Verification items for the finished model (mm, model axes). A direction names the side the tool comes from. Round coordinates to 2 decimals unless told otherwise and drop trailing zeros. Write each loop counter-clockwise with the first axis right and the second up, starting at its lowest first coordinate (ties: lowest second). Pieces come first, ordered by that corner, then holes. Notation, with made-up numbers: (40.25, -40) - (92.25, -40) arc R13 ccw to (92.25, -16) - close; hole circle Ø11 at (-38, -31). An arc over 180 degrees is marked (long way). Answer as a JSON object with one key per item and string values.
Autodesk Inventor part; units mm, degrees
ref_plane "YZ Plane" through (0, 0, 0) normal (1, 0, 0) x (0, 1, 0)
ref_plane "XZ Plane" through (0, 0, 0) normal (0, 1, 0) x (-1, 0, 0)
ref_plane "XY Plane" through (0, 0, 0) normal (0, 0, 1) x (1, 0, 0)
sketch "Sketch1" plane through (0, 0, 0) normal (0, 0, 1) x (1, 0, 0)
  arc A0 (6.3048, 12.5) -> (6.3048, -12.5) centre (0, 0) ccw
  arc A1 (193.6952, -12.5) -> (193.6952, 12.5) centre (200, 0) ccw
  line L0 (6.3048, 12.5) -> (193.6952, 12.5)
  line L1 (193.6952, -12.5) -> (6.3048, -12.5)
  dimension "d0" = 25
  dimension "d2" = 14
  dimension "d3" = 200
extrude "Extrusion1" add sketch "Sketch1" along normal blind 25
sketch "Sketch2" plane through (0, 0, 25) normal (0, 0, 1) x (1, 0, 0)
  arc A0 (6.3048, 12.5) -> (6.3048, -12.5) centre (0, 0) ccw
  arc A1 (193.6952, -12.5) -> (193.6952, 12.5) centre (200, 0) ccw
  circle A2 centre (0, 0) radius 11.05
  circle A3 centre (200, 0) radius 11.05
  dimension "d6" = 22.1
extrude "Extrusion2" cut sketch "Sketch2" against normal blind 7
sketch "Sketch3" plane through (0, 0, 0) normal (0, 0, -1) x (-1, 0, 0)
  circle A0 centre (-200, 0) radius 11.05
  circle A1 centre (0, 0) radius 11.05
extrude "Extrusion3" cut sketch "Sketch3" against normal blind 7
sketch "Sketch4" plane through (200, 0, 7) normal (0, 0, -1) x (-1, 0, 0)
  circle A0 centre (0, 0) radius 11.05
  circle A1 centre (200, 0) radius 11.05
  circle A2 centre (0, 0) radius 7.55
  circle A3 centre (200, 0) radius 7.55
  dimension "d12" = 15.1
extrude "Extrusion4" cut sketch "Sketch4" against normal through all contours A2 | A3
chamfer "Chamfer1" distance 3.5 angle 45 2 edges at (207.55, 0, 7) (7.55, 0, 7)
properties part number "ARM"
1. Cross-section at D-D (z = 13.75). Record the boundary of the cut face in (x, y), plus the area to 3 significant figures.
Completed:
{"outline": "(6.3, -12.5) - (193.7, -12.5) arc R14 ccw (long way) to (193.7, 12.5) - (6.3, 12.5) arc R14 ccw (long way) to start; hole circle Ø15.1 at (0, 0); hole circle Ø15.1 at (200, 0)", "area": "5,280 mm^2"}
2. Cross-section at C-C (z = 4.25). Record the boundary of the cut face in (x, y), plus the area to 3 significant figures.
Completed:
{"outline": "(6.3, -12.5) - (193.7, -12.5) arc R14 ccw (long way) to (193.7, 12.5) - (6.3, 12.5) arc R14 ccw (long way) to start; hole circle Ø22.1 at (0, 0); hole circle Ø22.1 at (200, 0)", "area": "4,870 mm^2"}
3. Access from +Z, -Z, +X, -X, +Y, -Y to the whole of each face (thin tool, end or side, straight path). Record for faces 3 (the face through (99, 12.5, 12)), 4 (the face through (2.395, -10.787, 3.451)), 5 (the face through (-2.395, -10.787, 21.549)), 6 (the face through (101, -12.5, 12)).
Completed:
{"face 3": "+Z, -Z, +Y", "face 4": "-Z", "face 5": "+Z", "face 6": "+Z, -Z, -Y"}
4. Material ranges on probe 1 along X at (y, z) = (-0.5, 6.75); probe 2 along Y at (x, z) = (0, 5.25); probe 3 along Y at (x, z) = (200, 12.5), recorded low to high. Write a range as from..to.
Completed:
{"probe 1": "x = -13.99..-11.04, 11.04..188.96, 211.04..213.99", "probe 2": "y = -14..-11.05, 11.05..14", "probe 3": "y = -14..-7.55, 7.55..14"}
5. Go/stop test with flat-tipped pins: pin 1 (3 mm diameter, centred on y = -9, z = 8, fed in from +X); pin 2 (1.5 mm diameter, centred on y = -2, z = 20.5, fed in from -X); pin 3 (11 mm diameter, centred on x = -2.5, y = -3, fed in from -Z). Record where each tip stops, or that it passes through.
Completed:
{"pin 1": "stops at x = 211.82", "pin 2": "stops at x = -13.94", "pin 3": "stops at z = 8.64"}
6. Mould release check, pull along X, two halves, no side actions. Record for faces 1 (the face through (1.684, -7.584, 10.281)), 2 (the face through (98, 0, 25)): released by +X, released by -X, zero draft, split by the parting line, or undercut.
Completed:
{"face 1": "undercut", "face 2": "zero draft"}
7. Cross-section at A-A (y = 0). Count the separate pieces of the cut face and the enclosed holes in it, plus the area to 3 significant figures.
Completed:
{"separate pieces": "3", "enclosed holes": "0", "area": "4,720 mm^2"}
